Read the model definition and answer for the solid it produces. Units are mm, in the model's axes. A direction names the side the tool comes from. Coordinates: 2 decimals unless noted, no trailing zeros. Write each loop counter-clockwise with the first axis right and the second up, starting at its lowest first coordinate (ties: lowest second). Pieces come first, ordered by that corner, then holes. Notation, with made-up numbers: (6, -27.5) - (44, -27.5) arc R13 ccw to (44, -3.5) - close; hole circle Ø2 at (87, 30). An arc over 180 degrees is marked (long way). Return JSON: item names as keys, results as strings.
```python
from build123d import *

# Parameters (mm, degrees)
SKETCH1_R           = 1.75
BOSS_EXTRUDE1_DEPTH = 2
FILLET3_SIZE        = 2
SKETCH2_R           = 1.75
SKETCH2_R_2         = 3
CUT_EXTRUDE1_DEPTH  = 60.602891692


with BuildPart() as part:
    # Sketch1 → Boss-Extrude1 (new body)
    with BuildSketch(Plane(origin=(0, 0, 0), x_dir=(1, 0, 0), z_dir=(0, 1, 0))):
        Polygon((12.5, -17.149645759), (24, -7.5), (54, -7.5), (54, 7.5), (24, 7.5), (12.5, 23.863068172), (-12.5, 23.863068172), (-32.938151944, 0), (-12.5, -17.149645759), (-12.5, -25.149645759), (12.5, -25.149645759), align=None)
        with Locations(Location((51.5, -5, 0), (0, 0, 270))):
            Circle(SKETCH1_R, mode=Mode.SUBTRACT)
        with Locations(Location((51.5, 5, 0), (0, 0, 90))):
            Circle(SKETCH1_R, mode=Mode.SUBTRACT)
        with BuildLine():
            Line((22.5, 4), (49.5, 4))
            Line((49.5, 4), (49.5, -4))
            Line((49.5, -4), (22.5, -4))
            ThreePointArc((22.5, -4), (6.5, 0), (22.5, 4))
        make_face(mode=Mode.SUBTRACT)
    extrude(amount=BOSS_EXTRUDE1_DEPTH)

    # Fillet2
    # a fillet whose section is not a circle: 21 mm, written as the material it takes off along each edge
    with BuildSketch(Plane(origin=(-32.938151944, -53.033486064, 0), x_dir=(0.650499477323288, 0, -0.7595067017493191), z_dir=(0, 1, 0))) as fillet2_piece_1:
        with BuildLine():
            Bezier((21.213394426, 0), (0, 0), (0.214467683, -21.212310262), weights=[1, 3, 1])
            Line((0.214467683, -21.212310262), (0, 0))
            Line((0, 0), (21.213394426, 0))
        make_face()
    extrude(amount=108.066972128, mode=Mode.SUBTRACT)

    # Fillet3
    # a fillet whose section is not a circle: 2 mm, written as the material it takes off along each edge
    with BuildSketch(Plane(origin=(54, -5, -7.5), x_dir=(0, 0, 1), z_dir=(0, 1, 0)), Plane(origin=(54, -5, 7.5), x_dir=(-1, 0, 0), z_dir=(0, 1, 0))) as fillet3_piece_1:
        with BuildLine():
            Bezier((FILLET3_SIZE, 0), (0, 0), (0, -FILLET3_SIZE), weights=[1, 3, 1])
            Line((0, -FILLET3_SIZE), (0, 0))
            Line((0, 0), (FILLET3_SIZE, 0))
        make_face()
    extrude(amount=12, mode=Mode.SUBTRACT)

    # Sketch2 → Cut-Extrude1 (cut, through all)
    with BuildSketch(Plane(origin=(0, 2, 0), x_dir=(1, 0, 0), z_dir=(0, 1, 0))):
        with Locations(Location((-9.5, -22.149645759, 0), (0, 0, 270))):
            Circle(SKETCH2_R)
        with Locations(Location((9.5, -22.149645759, 0), (0, 0, 270))):
            Circle(SKETCH2_R)
        with Locations(Location((6, 20.363068172, 0), (0, 0, 270))):
            Circle(SKETCH2_R)
        with Locations(Location((-6, 20.363068172, 0), (0, 0, 270))):
            Circle(SKETCH2_R)
        with Locations(Location((0, -15.149645759, 0), (0, 0, 270))):
            Circle(SKETCH2_R)
        with Locations(Location((-17.5, 0, 0), (0, 0, 270))):
            Circle(SKETCH2_R)
        with Locations(Location((1.200212435, 4.853811915, 0), (0, 0, 270))):
            Circle(SKETCH2_R)
        with Locations(Location((0, 13.363068172, 0), (0, 0, 270))):
            Circle(SKETCH2_R_2)
        with Locations(Location((1.2, -5, 0), (0, 0, 270))):
            Circle(SKETCH2_R)
        with BuildLine():
            Line((-5.5, 6), (-5.5, -6))
            ThreePointArc((-5.5, -6), (-9.5, -10), (-13.5, -6))
            Line((-13.5, -6), (-13.5, 6))
            ThreePointArc((-13.5, 6), (-9.5, 10), (-5.5, 6))
        make_face()
    extrude(amount=-CUT_EXTRUDE1_DEPTH, mode=Mode.SUBTRACT)


solid = part.part
```
(1) A cutting plane is placed at C-C (z = 19). Determine the outline of the cut face in (x, y).
Answer:
{"outline": "(-12.5, 0) - (12.5, 0) - (12.5, 2) - (-12.5, 2) - close"}
(2) Determine the mould class of faces 1 (the face through (-12.5, 1, 21)), 2 (the face through (-0.67, 1.014, 16.766)), 3 (the face through (0, 1, 25.15)) for opening direction X: +X half, -X half, draft (parallel to the pull), parting line (faces both ways), or undercut.
Answer:
{"face 1": "-X half", "face 2": "undercut", "face 3": "draft"}
(3) A cutting plane is placed at A-A (x = 29). Determine the outline of the cut face in (y, z), and give its area (3 significant figures).
Answer:
{"outline": "(0, -7.5) - (2, -7.5) - (2, -4) - (0, -4) - close; (0, 4) - (2, 4) - (2, 7.5) - (0, 7.5) - close", "area": "14.0 mm²"}
(4) A cutting plane is placed at D-D (y = 0.5). State how many separate pieces and enclosed holes the cut face has, and give its area (3 significant figures).
Answer:
{"separate pieces": "1", "enclosed holes": "13", "area": "1,680 mm²"}
(5) Which of the six approach directions +Z, -Z, +X, -X, +Y, -Y give full straight-line access (tool end or side, diameter ignored) to faces 4 (the face through (0, 1, -23.863)), 5 (the face through (-13.5, 1, 0)), 6 (the face through (38, 1, -7.5))?
Answer:
{"face 4": "-Z, +X, -X, +Y, -Y", "face 5": "+Y, -Y", "face 6": "-Z, +X, +Y, -Y"}
(6) Flat-ended cylindrical pins translate along their axes: P1, Ø1.5, axis at x = 24.5, z = 10.5, coming from the +Y side; P2, Ø1, axis at x = 34.5, y = 1, coming from the +Z side; P3, Ø0.6, axis at y = 0.5, z = 19.5, coming from the +X side. Find the tip coordinate at first contact, or state that the pin passes through.
Answer:
{"P1": "through", "P2": "z = 7.5", "P3": "x = 12.5"}
(7) Straight lines are drawn through the part: line 1 (Z direction, x = 33, y = 1.45); line 2 (X direction, y = 0.7, z = 21); line 3 (X direction, y = 0.9, z = -6). For each, find the intervals that lie inside material, in ascending order. Write a range as from..to.
Answer:
{"line 1": "-7.5..-4, 4..7.5", "line 2": "-12.5..-10.82, -8.18..8.18, 10.82..12.5", "line 3": "-27.13..-13.5, -5.5..-0.12, 2.52..8.98, 21.02..50.06, 52.94..54"}
(8) A cutting plane is placed at B-B (x = 9.5). Determine the outline of the cut face in (y, z), and give its area (3 significant figures).
Answer:
{"outline": "(0, -23.86) - (2, -23.86) - (2, -6.48) - (0, -6.48) - close; (0, 6.48) - (2, 6.48) - (2, 20.4) - (0, 20.4) - close; (0, 23.9) - (2, 23.9) - (2, 25.15) - (0, 25.15) - close", "area": "65.1 mm²"}
